The listing builds one solid part. Answer for the finished solid, in the listing's coordinates (mm). A direction names the side the tool comes from. Give positions to 0.01 mm unless a question says otherwise; leave off trailing zeros. Loops run counter-clockwise (first coordinate to the right, second up) from the corner with the lowest first, then second, coordinate; pieces in that order, holes last. Notation, with made-up numbers: (-20.75, 73) - (33.25, 73) arc R29 cw to (33.25, 103) - close; hole circle Ø6 at (-37.5, 33). An arc over 180 degrees is marked (long way). Write item = value, one per line. Start each with the question number.
1) Flat-ended cylindrical pins translate along their axes: P1, Ø5, axis at x = -18, z = 5, coming from the +Y side; P2, Ø0.8, axis at y = 6, z = 6.5, coming from the -X side; P3, Ø2.5, axis at y = 1.5, z = 16.5, coming from the -X side. Find the tip coordinate at first contact, or state that the pin passes through.
2) The mould has two halves that part along Y. Classify faces 1 (the flat face through (-4, 0, 17)), 2 (the flat face through (-19, 5, 5)), 3 (the flat face through (-5, 2, 0)): +Y half, -Y half, draft (parallel to the pull), parting line (faces both ways), or undercut.
3) Consider probe 1 along Y at (x, z) = (-17, 7.5); probe 2 along X at (y, z) = (-0.25, 2.75); probe 3 along Y at (x, z) = (-10.5, 22.75). Determine where each line is inside the solid, lowest interval first.
4) The part is cut by section A-A on z = 3.25. Write down the section's boundary in (x, y).
5) The part is cut by section C-C on z = 14.25. Write down the section's boundary in (x, y), plus the area to 3 significant figures.
6) The part is cut by section B-B on x = -13. Write down the section's boundary in (y, z), plus the area to 3 significant figures.
7) Which of the six approach directions +Z, -Z, +X, -X, +Y, -Y give full straight-line access (tool end or side, diameter ignored) to faces 4 (the flat face through (-13, 3, 10)), 5 (the flat face through (-12.5, 6, 12)), 6 (the flat face through (-16, 0, 5))?
from build123d import *

# Parameters (mm, degrees)
F0_W     = 12.5
F0_H     = 2.5
F1_DEPTH = 25
F2_R     = 1
F3_DEPTH = 10


with BuildPart() as f1:
    # F0 (on Top) → F1 (new body)
    with BuildSketch(Plane.XY):
        with BuildLine():
            Line((0, 7.5), (0, 5))
            Line((0, 5), (0, 0))
            Line((0, 0), (-7.5, 0))
            ThreePointArc((-7.5, 0), (0, -7.5), (7.5, 0))
            ThreePointArc((7.5, 0), (5.3033008589, 5.3033008589), (0, 7.5))
        make_face()
        with Locations((-6.25, 6.25)):
            Rectangle(F0_W, F0_H)
    extrude(amount=F1_DEPTH)

    # F2
    f2_edges = [f1.edges().sort_by_distance(p)[0] for p in [
        (-6.25, 7.5, 25),
        (-12.5, 6.25, 25),
        (-6.25, 5, 25),
        (0, 2.5, 25),
        (-3.75, 0, 25),
        (5.303301, -5.303301, 25),
    ]]
    fillet(f2_edges, radius=F2_R)

    # F0 (on Top) → F3 (join)
    with BuildSketch(Plane.XY):
        Polygon((0, 5), (-12.5, 5), (-12.5, 0), (-7.5, 0), (0, 0), align=None)
        with BuildLine():
            Line((-12.5, 0), (-12.5, 5))
            ThreePointArc((-12.5, 5), (-16.0355339059, 3.5355339059), (-17.5, 0))
            Line((-17.5, 0), (-12.5, 0))
        make_face()
        with BuildLine():
            ThreePointArc((-17.5, 0), (-16.0355339059, 3.5355339059), (-12.5, 5))
            Line((-12.5, 5), (-25, 5))
            Line((-25, 5), (-25, 0))
            Line((-25, 0), (-17.5, 0))
        make_face()
    extrude(amount=F3_DEPTH)


solid = f1.part
Answer below:
q1.P1 = 5
q1.P2 = -12.5
q1.P3 = 0
q2.face_1 = undercut
q2.face_2 = +Y half
q2.face_3 = draft
q3.probe_1 = 0 to 5
q3.probe_2 = -7.5 to 7.5
q3.probe_3 = 5 to 7.5
q4.outline = (-25, 0) - (-7.5, 0) arc R7.5 ccw (long way) to (0, 7.5) - (-12.5, 7.5) - (-12.5, 5) - (-25, 5) - close
q5.outline = (-12.5, 5) - (0, 5) - (0, 0) - (-7.5, 0) arc R7.5 ccw (long way) to (0, 7.5) - (-12.5, 7.5) - close
q5.area = 164 mm2
q6.outline = (0, 0) - (5, 0) - (5, 10) - (0, 10) - close
q6.area = 50.0 mm2
q7.face_4 = +Z, -X
q7.face_5 = +Z, -Z, -X, +Y
q7.face_6 = +Z, -Z, -X, -Y
